Source: CAD feature listing. Evaluate the final solid. Frame: model axes, mm. A direction names the side the tool comes from. Round coordinates to 2 decimals unless told otherwise and drop trailing zeros. Loops run counter-clockwise (first coordinate to the right, second up) from the corner with the lowest first, then second, coordinate; pieces in that order, holes last.
Item 1: Section query A-A on z = 6. Return loops of the section in (x, y).
Item 2: Ray query, L1, parallel to Y at x = -4, z = 5; L2, parallel to X at y = 6.5, z = 6; L3, parallel to Y at x = 7.5, z = 3. Return the intervals inside material, ascending.
Item 3: Access query for faces 1 (the flat face through (-13, 34, 0)), 2 (the cylindrical face through (-39.597, 25.68, 6.261)). Directions: +Z, -Z, +X, -X, +Y, -Y. A direction counts if a zero-diameter tool reaches every point of the face in a straight line with its end or side. Return the directions, or none.
Item 4: First-contact query: P1, Ø5, axis at y = 53.5, z = 7.5, coming from the -X side; P2, Ø6, axis at x = -31.5, z = 10.5, coming from the +Y side; P3, Ø5, axis at y = 25, z = 9.5, coming from the -X side. Flat tips, straight axial feed; report the tip coordinate or a pass-through.
Item 5: Pull-direction query (Y, two-part tool) for faces 3 (the cylindrical face through (12.41, 56.56, 6.26)), 4 (the flat face through (-13, 34, 12.7)); classes: released by +Y, released by -Y, zero draft, split by the parting line, or undercut.
Item 6: Section query B-B on x = 12.5. Give the number of separate pieces and of enclosed holes in the cut face, then the cut area to 3 significant figures.
```python
from build123d import *

# Parameters (mm, degrees)
F1_DEPTH = 12.7
F2_R     = 5.07999


# Not quite as in the source:
# - a fillet or chamfer is up to 0.001 mm smaller than in the source, because OpenCascade refuses the exact size


with BuildPart() as f1:
    # F0 (on Top) → F1 (new body)
    with BuildSketch(Plane.XY):
        with BuildLine():
            ThreePointArc((-27.1257893014, 52.8568671478), (-22.1396459711, 56.3482022942), (-16.6229893761, 58.9206615119))
            Line((-16.6229893761, 58.9206615119), (-18.3604517042, 63.6943000255))
            ThreePointArc((-18.3604517042, 63.6943000255), (-24.6796459711, 60.7476113455), (-30.3911503586, 56.7483729188))
            Line((-30.3911503586, 56.7483729188), (-27.1257893014, 52.8568671478))
        make_face()
        with BuildLine():
            ThreePointArc((-27.1257893014, -0.6436767596), (-39.5996459711, 26.1065951941), (-27.1257893014, 52.8568671478))
            Line((-27.1257893014, 52.8568671478), (-30.3911503586, 56.7483729188))
            ThreePointArc((-30.3911503586, 56.7483729188), (-44.6796459711, 26.1065951941), (-30.3911503586, -4.5351825307))
            Line((-30.3911503586, -4.5351825307), (-27.1257893014, -0.6436767596))
        make_face()
        with BuildLine():
            Line((-18.3604517042, -11.4811096374), (-16.6229893761, -6.7074711238))
            ThreePointArc((-16.6229893761, -6.7074711238), (-22.1396459711, -4.1350119061), (-27.1257893014, -0.6436767596))
            Line((-27.1257893014, -0.6436767596), (-30.3911503586, -4.5351825307))
            ThreePointArc((-30.3911503586, -4.5351825307), (-24.6796459711, -8.5344209573), (-18.3604517042, -11.4811096374))
        make_face()
        with BuildLine():
            Line((34.7126641494, 19.1606680874), (29.709840764, 20.04280083))
            ThreePointArc((29.709840764, 20.04280083), (12.7803540289, -4.1350119061), (-16.6229893761, -6.7074711238))
            Line((-16.6229893761, -6.7074711238), (-18.3604517042, -11.4811096374))
            ThreePointArc((-18.3604517042, -11.4811096374), (15.3203540289, -8.5344209573), (34.7126641494, 19.1606680874))
        make_face()
        with BuildLine():
            Line((34.7126641494, 33.0525223008), (29.709840764, 32.1703895582))
            ThreePointArc((29.709840764, 32.1703895582), (30.1074728862, 29.1500737308), (30.2403540289, 26.1065951941))
            ThreePointArc((30.2403540289, 26.1065951941), (30.1074728862, 23.0631166573), (29.709840764, 20.04280083))
            Line((29.709840764, 20.04280083), (34.7126641494, 19.1606680874))
            ThreePointArc((34.7126641494, 19.1606680874), (35.1681419525, 22.6203654842), (35.3203540289, 26.1065951941))
            ThreePointArc((35.3203540289, 26.1065951941), (35.1681419525, 29.592824904), (34.7126641494, 33.0525223008))
        make_face()
        with BuildLine():
            ThreePointArc((-15.0156707349, 38.4245898394), (-12.7196459711, 40.0322836869), (-10.1793298758, 41.2168525363))
            Line((-10.1793298758, 41.2168525363), (-16.6229893761, 58.9206615119))
            ThreePointArc((-16.6229893761, 58.9206615119), (-22.1396459711, 56.3482022942), (-27.1257893014, 52.8568671478))
            Line((-27.1257893014, 52.8568671478), (-15.0156707349, 38.4245898394))
        make_face()
        with BuildLine():
            ThreePointArc((-8.4418675477, 36.4432140227), (0.8203540289, 35.6328746357), (6.153239312, 28.0167251484))
            Line((6.153239312, 28.0167251484), (11.1560626973, 28.898857891))
            ThreePointArc((11.1560626973, 28.898857891), (3.3603540289, 40.0322836869), (-10.1793298758, 41.2168525363))
            Line((-10.1793298758, 41.2168525363), (-8.4418675477, 36.4432140227))
        make_face()
        with BuildLine():
            ThreePointArc((-11.7503096777, 17.6801063198), (-15.6796459711, 26.1065951941), (-11.7503096777, 34.5330840684))
            Line((-11.7503096777, 34.5330840684), (-15.0156707349, 38.4245898394))
            ThreePointArc((-15.0156707349, 38.4245898394), (-20.7596459711, 26.1065951941), (-15.0156707349, 13.7886005487))
            Line((-15.0156707349, 13.7886005487), (-11.7503096777, 17.6801063198))
        make_face()
        with BuildLine():
            ThreePointArc((-11.7503096777, 34.5330840684), (-10.1796459711, 35.6328746357), (-8.4418675477, 36.4432140227))
            Line((-8.4418675477, 36.4432140227), (-10.1793298758, 41.2168525363))
            ThreePointArc((-10.1793298758, 41.2168525363), (-12.7196459711, 40.0322836869), (-15.0156707349, 38.4245898394))
            Line((-15.0156707349, 38.4245898394), (-11.7503096777, 34.5330840684))
        make_face()
        with BuildLine():
            Line((11.1560626973, 23.3143324972), (6.153239312, 24.1964652397))
            ThreePointArc((6.153239312, 24.1964652397), (0.8203540289, 16.5803157525), (-8.4418675477, 15.7699763654))
            Line((-8.4418675477, 15.7699763654), (-10.1793298758, 10.9963378518))
            ThreePointArc((-10.1793298758, 10.9963378518), (3.3603540289, 12.1809067012), (11.1560626973, 23.3143324972))
        make_face()
        with BuildLine():
            ThreePointArc((6.153239312, 28.0167251484), (6.2784957079, 27.0653083643), (6.3203540289, 26.1065951941))
            ThreePointArc((6.3203540289, 26.1065951941), (6.2784957079, 25.1478820239), (6.153239312, 24.1964652397))
            Line((6.153239312, 24.1964652397), (11.1560626973, 23.3143324972))
            ThreePointArc((11.1560626973, 23.3143324972), (11.3391647742, 24.7051308507), (11.4003540289, 26.1065951941))
            ThreePointArc((11.4003540289, 26.1065951941), (11.3391647742, 27.5080595375), (11.1560626973, 28.898857891))
            Line((11.1560626973, 28.898857891), (6.153239312, 28.0167251484))
        make_face()
        with BuildLine():
            Line((-10.1793298758, 10.9963378518), (-8.4418675477, 15.7699763654))
            ThreePointArc((-8.4418675477, 15.7699763654), (-10.1796459711, 16.5803157525), (-11.7503096777, 17.6801063198))
            Line((-11.7503096777, 17.6801063198), (-15.0156707349, 13.7886005487))
            ThreePointArc((-15.0156707349, 13.7886005487), (-12.7196459711, 12.1809067012), (-10.1793298758, 10.9963378518))
        make_face()
        with BuildLine():
            ThreePointArc((-16.6229893761, 58.9206615119), (12.7803540289, 56.3482022942), (29.709840764, 32.1703895582))
            Line((29.709840764, 32.1703895582), (34.7126641494, 33.0525223008))
            ThreePointArc((34.7126641494, 33.0525223008), (15.3203540289, 60.7476113455), (-18.3604517042, 63.6943000255))
            Line((-18.3604517042, 63.6943000255), (-16.6229893761, 58.9206615119))
        make_face()
        with BuildLine():
            Line((29.709840764, 32.1703895582), (11.1560626973, 28.898857891))
            ThreePointArc((11.1560626973, 28.898857891), (11.3391647742, 27.5080595375), (11.4003540289, 26.1065951941))
            ThreePointArc((11.4003540289, 26.1065951941), (11.3391647742, 24.7051308507), (11.1560626973, 23.3143324972))
            Line((11.1560626973, 23.3143324972), (29.709840764, 20.04280083))
            ThreePointArc((29.709840764, 20.04280083), (30.1074728862, 23.0631166573), (30.2403540289, 26.1065951941))
            ThreePointArc((30.2403540289, 26.1065951941), (30.1074728862, 29.1500737308), (29.709840764, 32.1703895582))
        make_face()
        with BuildLine():
            Line((-16.6229893761, -6.7074711238), (-10.1793298758, 10.9963378518))
            ThreePointArc((-10.1793298758, 10.9963378518), (-12.7196459711, 12.1809067012), (-15.0156707349, 13.7886005487))
            Line((-15.0156707349, 13.7886005487), (-27.1257893014, -0.6436767596))
            ThreePointArc((-27.1257893014, -0.6436767596), (-22.1396459711, -4.1350119061), (-16.6229893761, -6.7074711238))
        make_face()
    extrude(amount=F1_DEPTH)

    # F2 (radius 5.08 in the source; OpenCascade refuses exactly that, so slightly less here)
    f2_edges = [f1.edges().sort_by_distance(p)[0] for p in [
        (-44.071956, 19.160668, 12.7),
        (-44.071956, 19.160668, 0),
    ]]
    fillet(f2_edges, radius=F2_R)


solid = f1.part
```
Data:
1. outline: circle Ø80 at (-4.68, 26.11); hole (-27.13, -0.64) - (-15.02, 13.79) arc R16.08 cw to (-15.02, 38.42) - (-27.13, 52.86) arc R34.92 ccw to start; hole (-16.62, -6.71) arc R34.92 ccw to (29.71, 20.04) - (11.16, 23.31) arc R16.08 cw to (-10.18, 11) - close; hole (-16.62, 58.92) - (-10.18, 41.22) arc R16.08 cw to (11.16, 28.9) - (29.71, 32.17) arc R34.92 ccw to start; hole circle Ø22 at (-4.68, 26.11)
2. L1: y = -13.89 to -8.81, 10.04 to 15.13, 37.09 to 42.17, 61.02 to 66.1
2. L2: x = -39.54 to -33.58, -21.13 to -11.82, 24.22 to 30.19
2. L3: y = -11.53 to -6.62, 15.61 to 36.61, 58.83 to 63.74
3. face 1: -Z, +X, -X, +Y, -Y
3. face 2: +Z, -Z
4. P1: stops at x = -35.99
4. P2: stops at y = 57.7
4. P3: stops at x = -44.68
5. face 3: undercut
5. face 4: zero draft
6. separate pieces: 3
6. enclosed holes: 0
6. area: 198 mm2
